from build123d import *

# Parameters (mm, degrees)
F0_W     = 762
F0_H     = 457.2
F0_R     = 142.875
F1_DEPTH = 38.1
F2_R     = 12.7
F3_R     = 5.08


with BuildPart() as f1:
    # F0 (on Front) → F1 (new body)
    with BuildSketch(Plane.XZ):
        Rectangle(F0_W, F0_H)
        with Locations((-186.950803, 0)):
            Circle(F0_R, mode=Mode.SUBTRACT)
        with Locations((188.911736, 0)):
            Circle(F0_R, mode=Mode.SUBTRACT)
    extrude(amount=F1_DEPTH)

    # F2
    f2_edges = [f1.edges().sort_by_distance(p)[0] for p in [
        (0, -38.1, 228.6),
        (0, -38.1, -228.6),
    ]]
    fillet(f2_edges, radius=F2_R)

    # F3
    f3_edges = [f1.edges().sort_by_distance(p)[0] for p in [
        (-329.825803, -38.1, 0),
        (46.036736, -38.1, 0),
    ]]
    fillet(f3_edges, radius=F3_R)


solid = f1.part
Model file for the job. Use its own axes, mm. Coordinates: 2 decimals unless noted, no trailing zeros. Order: outer loops, then holes, each group sorted by start corner. A loop starts at its lowest first (then second) coordinate and runs counter-clockwise, first axis right, second up. Notation, with made-up numbers: (-20, 50) -> (15, 50) arc R27 cw to (15, 68) -> close; hole circle Ø4 at (10.5, 45). An arc over 180 degrees is marked (long way). Return JSON: item names as keys, results as strings. Group by question number.
Item 1: Saw through at A-A on z = 0. Write the cut outline in (x, y).
Item 2: Flat gauge pin, fed straight in: P1, Ø1, axis at x = -185, y = -30, coming from the -Z side. Where does the tip first touch, or does it go through?
Item 3: Saw through at B-B on y = -18.5. Write the cut outline in (x, z) (3 decimals), then the cut area to 3 significant figures.
Item 4: Pull direction X, two halves, no side cores. Call faces 1 (the flat face through (-5, -13, -228.6)), 2 (the flat face through (-381, -19, -3)), 3 (the cylindrical face through (-50.674, -16.279, 42.916)), 4 (the flat face through (381, -19, -3)): pulls with the +X half, pulls with the -X half, needs draft (parallel to the pull), parting line crosses it, or undercut.
Item 5: Saw through at C-C on z = 97. State how many separate pieces and enclosed holes the cut face has, then the cut area to 3 significant figures.
Item 6: Wall check: line 1 along X through (y, z) = (-24, -1.5); line 2 along X through (y, z) = (-32, -32); line 3 along Z through (x, y) = (-312, -22). Give the ranges that are in metal, low to high. Write a range as [from, to].
Values found:
{
 "1": {"outline": "(-381, -38.1) -> (-334.91, -38.1) arc R5.08 ccw to (-329.83, -33.02) -> (-329.83, 0) -> (-381, 0) -> close; (-44.08, -33.02) arc R5.08 ccw to (-39, -38.1) -> (40.96, -38.1) arc R5.08 ccw to (46.04, -33.02) -> (46.04, 0) -> (-44.08, 0) -> close; (331.79, -33.02) arc R5.08 ccw to (336.87, -38.1) -> (381, -38.1) -> (381, 0) -> (331.79, 0) -> close"},
 "2": {"P1": "stops at z = -227.92"},
 "3": {"outline": "(-381, -228.6) -> (381, -228.6) -> (381, 228.6) -> (-381, 228.6) -> close; hole circle Ø285.75 at (-186.951, 0); hole circle Ø285.75 at (188.912, 0)", "area": "220,000 mm2"},
 "4": {"face 1": "needs draft", "face 2": "pulls with the -X half", "face 3": "undercut", "face 4": "pulls with the +X half"},
 "5": {"separate pieces": "3", "enclosed holes": "0", "area": "13,000 mm2"},
 "6": {"line 1": "x = [-381, -329.82], [-44.08, 46.04], [331.78, 381]", "line 2": "x = [-381, -326.2], [-47.71, 49.67], [328.16, 381]", "line 3": "z = [-228.6, -69.11], [69.11, 228.6]"}
}
